Autodesk Inventor part; units mm, degrees
ref_plane "YZ Plane" through (0, 0, 0) normal (1, 0, 0) x (0, 1, 0)
ref_plane "XZ Plane" through (0, 0, 0) normal (0, 1, 0) x (-1, 0, 0)
ref_plane "XY Plane" through (0, 0, 0) normal (0, 0, 1) x (1, 0, 0)
sketch "Sketch1" plane through (0, 0, 0) normal (0, 1, 0) x (-1, 0, 0)
  line L0 (0, 0) -> (8, 0)
  line L1 (8, 0) -> (8, -80)
  line L2 (0, -80) -> (0, 0)
  line L3 (8, -80) -> (57.5929, -216.2554)
  line L4 (8, -80) -> (153, -80) construction
  line L5 (57.5929, -216.2554) -> (50.0754, -218.9916)
  line L6 (50.0754, -218.9916) -> (0.4825, -82.7362)
  line L7 (0.4825, -82.7362) -> (0, -81.4106)
  line L8 (0, -81.4106) -> (0, -80)
  dimension "d3" = 8
  dimension "d4" = 80
  dimension "d6" = 70
  dimension "d7" = 8
extrude "Extrusion1" add sketch "Sketch1" along normal blind 8
sketch "Sketch2" plane through (-8, 0, 0) normal (0, 0, 1) x (1, 0, 0)
  line L0 (8, 8) -> (8, 15)
  line L1 (8, 8) -> (0, 8)
  line L2 (8, 8) -> (-42.0754, 8)
  line L3 (0, 8) -> (0, 15)
  line L4 (0, 15) -> (8, 15)
  point P0 (8, 0)
  dimension "d10" = 7
  dimension "d11" = 8
extrude "Extrusion2" add sketch "Sketch2" against normal blind 80
sketch "Sketch3" plane through (-57.5929, 0, -216.2554) normal (-0.342, 0, -0.9397) x (-0.9397, 0, 0.342)
  line L0 (-8, 0) -> (-8, 8)
  line L1 (0, 0) -> (0, 8)
  line L2 (-8, 8) -> (0, 8)
  line L3 (-7.5175, 15) -> (-7.5175, 8)
  line L4 (-8, 8) -> (-8, 15)
  line L5 (0, 8) -> (0, 15)
  line L6 (0, 15) -> (-8, 15)
  point P0 (19.8441, 0)
  dimension "d14" = 8
extrude "Extrusion3" add sketch "Sketch3" against normal blind 145
sketch "Sketch8" plane through (0, 0, 0) normal (0, -1, 0) x (1, 0, 0)
  line L0 (-8, -80) -> (-8, 0)
  line L1 (-8, -80) -> (0, -80)
  line L2 (0, -80) -> (0, -104)
  line L3 (0, -104) -> (-8, -104)
  line L4 (-8, -104) -> (-8, -80)
  circle A0 centre (-4, -100) radius 2.2
  circle A1 centre (-4, -84) radius 2.2
  point P0 (0, 0)
  point P1 (-4, -80)
  point P2 (-4, -104)
  dimension "d24" = 24
  dimension "d25" = 4.4
  dimension "d26" = 4.4
  dimension "d27" = 4
  dimension "d28" = 4
extrude "Extrusion7" add sketch "Sketch8" against normal blind 10
sketch "Sketch9" plane through (0, 10, 0) normal (0, 1, 0) x (1, 0, 0)
  line L0 (0, 80) -> (0, 104)
  line L1 (-8, 80) -> (-0.4825, 82.7362)
  line L2 (0, 104) -> (-8, 104)
  line L3 (-8, 104) -> (-8, 80)
  line L4 (-8, 80) -> (0, 80)
  line L5 (0, 80) -> (0, 104)
  point P0 (0, 0)
extrude "Extrusion8" cut sketch "Sketch9" along normal blind 145
extrude "Extrusion9" cut sketch "Sketch8" against normal blind 24 contours A1
chamfer "Chamfer1" distance 7 angle 84 1 edges at (-4, 15, 0) measured on face at (-5.3333, 5, 0)
chamfer "Chamfer2" distance 7 angle 75 1 edges at (-53.8342, 15, -217.6235) measured on face at (-55.0871, 5, -217.1675)
sketch "Sketch10" plane through (0, 10, 0) normal (0, 1, 0) x (1, 0, 0)
  line L0 (-8, 104) -> (0, 104)
  line L1 (-8, 104) -> (-8, 103.3904)
  line L2 (0, 104) -> (-8, 104)
  line L3 (-8, 104) -> (-8, 103.3904)
  line L4 (-8, 103.3904) -> (0, 103.3904)
  line L5 (0, 103.3904) -> (0, 104)
  point P0 (0, 0)
extrude "Extrusion10" cut sketch "Sketch10" against normal blind 10
properties part number "intake arm left"
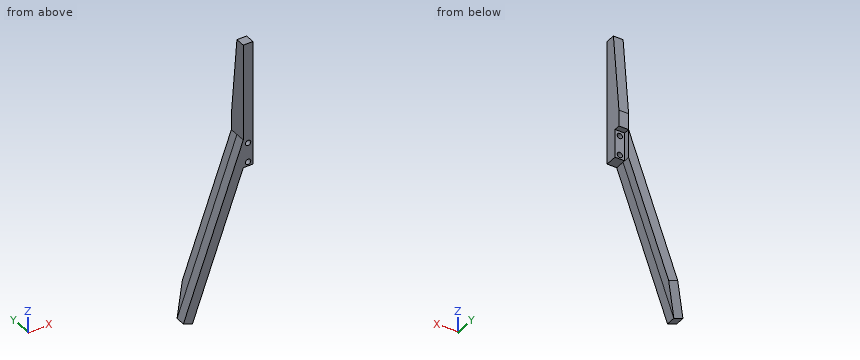
For this review, take the finished solid that the model builds, in its own axes (mm). Round coordinates to 2 decimals unless told otherwise and drop trailing zeros. Loops run counter-clockwise (first coordinate to the right, second up) from the corner with the lowest first, then second, coordinate; pieces in that order, holes last.
Q1. Insertion check: pin 1 Ø8 at (x, y) = (-46.5, 6) entering from -Z; pin 2 Ø2.5 at (x, y) = (-5.5, 4) entering from -Z; pin 3 Ø7 at (x, z) = (-4, -84) entering from +Y; pin 4 Ø6 at (x, z) = (-12.5, -30.5) entering from +Y. Each pin has a flat end and moves straight along its axis. Give the tip position at first contact, or say it passes through.
Result sheet:
pin 1: stops at z = -218.99
pin 2: stops at z = -103.39
pin 3: stops at y = 10
pin 4: passes through
Q2. Add section A-A on x = -4. Write out the cut boundary in (y, z), plus the area to 3 significant figures.
Result sheet:
outline: (0, -103.39) - (10, -103.39) - (10, -102.2) - (0, -102.2) - close; (0, -97.8) - (10, -97.8) - (10, -86.2) - (0, -86.2) - close; (0, -81.8) - (10, -81.8) - (10, -80) - (15, -80) - (15, -66.6) - (8, 0) - (0, 0) - close
area: 1,110 mm2
Q3. To check wall thickness, follow line 1 along Z through (x, y) = (-4, 3.5); line 2 along Z through (x, y) = (-5.5, 7.75); line 3 along X through (y, z) = (1, -12.5). State the ranges of each line that lie inside material, in increasing order.
Result sheet:
line 1: z = -103.39 to -102.2, -97.8 to -86.2, -81.8 to 0
line 2: z = -103.39 to -101.61, -98.39 to -85.61, -82.39 to 0
line 3: x = -8 to 0
Q4. Add section B-B on z = -100. Write out the cut boundary in (x, y), plus the area to 3 significant figures.
Result sheet:
outline: (-15.28, 0) - (-6.2, 0) - (-6.2, 10) - (-8, 10) - (-8, 15) - (-15.28, 15) - close; (-1.8, 0) - (0, 0) - (0, 10) - (-1.8, 10) - close
area: 145 mm2
Q5. Add section C-C on y = 5. Give the number of separate pieces and of enclosed holes in the cut face, plus the area to 3 significant figures.
Result sheet:
separate pieces: 1
enclosed holes: 2
area: 1,870 mm2
